The listing builds one solid part. Answer for the finished solid, in the listing's coordinates (mm). Face numbers are marked on the shaded views. A direction names the side the tool comes from. Coordinates: 2 decimals unless noted, no trailing zeros. Loops run counter-clockwise (first coordinate to the right, second up) from the corner with the lowest first, then second, coordinate; pieces in that order, holes last. Notation, with made-up numbers: M 6,-18 L 24,-18 A33 cw 24,11 Z; hole C -17,55.25 d6. An arc over 180 degrees is marked long. Answer in a Markdown table with one row per item. Add a question column.
from build123d import *

# Parameters (mm, degrees)
SKETCH001_W  = 155
SKETCH001_H  = 210
PAD_DEPTH    = 25
THICKNESS_T  = -0.5
SKETCH_W     = 30
SKETCH_H     = 13.5
PAD001_DEPTH = 5
FILLET_R     = 1
FILLET001_R  = 1


with BuildPart() as part:
    # Sketch001 → Pad (new body)
    with BuildSketch(Plane.XY):
        with Locations((77.5, 105)):
            Rectangle(SKETCH001_W, SKETCH001_H)
    extrude(amount=PAD_DEPTH)

    # Thickness
    thickness_openings = [part.faces().sort_by_distance(p)[0] for p in [
        (77.5, 105, 25),
    ]]
    offset(amount=THICKNESS_T, openings=thickness_openings)

    # Sketch → Pad001 (join)
    with BuildSketch(Plane.XY):
        with Locations((50, 105)):
            Rectangle(SKETCH_W, SKETCH_H)
        with Locations((105, 105)):
            Rectangle(SKETCH_W, SKETCH_H)
    extrude(amount=PAD001_DEPTH)

    # Fillet
    fillet_edges = [part.edges().sort_by_distance(p)[0] for p in [
        (77.5, 0.5, 0.5),
        (0.5, 105, 0.5),
        (154.5, 105, 0.5),
        (77.5, 209.5, 0.5),
        (50, 98.25, 0.5),
        (65, 105, 0.5),
        (50, 111.75, 0.5),
        (35, 105, 0.5),
        (120, 105, 0.5),
        (105, 111.75, 0.5),
        (90, 105, 0.5),
        (105, 98.25, 0.5),
    ]]
    fillet(fillet_edges, radius=FILLET_R)

    # Fillet001
    fillet001_edges = [part.edges().sort_by_distance(p)[0] for p in [
        (35, 105, 5),
        (50, 98.25, 5),
        (65, 105, 5),
        (50, 111.75, 5),
        (120, 105, 5),
        (105, 98.25, 5),
        (90, 105, 5),
        (105, 111.75, 5),
    ]]
    fillet(fillet001_edges, radius=FILLET001_R)


solid = part.part
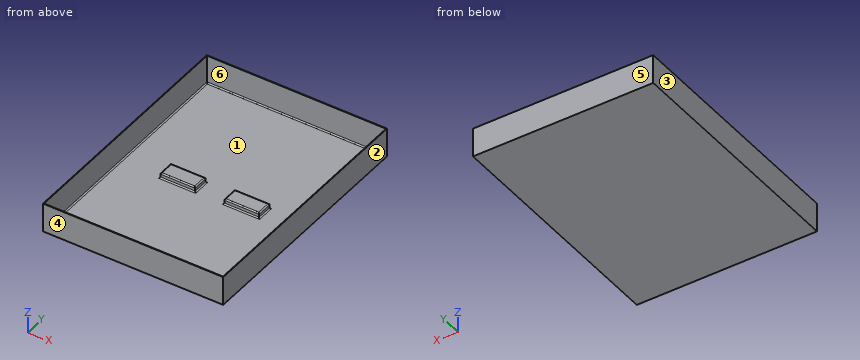
(1) Straight lines are drawn through the part: line 1 (X direction, y = 81, z = 2.5); line 2 (Y direction, x = 143, z = 10); line 3 (Z direction, x = 68, y = 117). For each, find the intervals that lie inside material, in ascending order.
(2) A cutting plane is placed at A-A (x = 47). Give the vertices of the cut face in (y, z).
(3) A cutting plane is placed at B-B (y = 108). Give the vertices of the cut face in (x, z), plus the area to 3 significant figures.
(4) A cutting plane is placed at D-D (x = 130). Give the vertices of the cut face in (y, z), plus the area to 3 significant figures.
(5) The mould has two halves that part along X. Classify the marked faces 1, 2, 3 and 4: released by +X, released by -X, zero draft, split by the parting line, or undercut.
(6) A cutting plane is placed at C-C (z = 13). Give the vertices of the cut face in (x, y).
(7) For the marked faces 5 and 6, determine the directions among +Z, -Z, +X, -X, +Y, -Y from which every point of the face is accessible in a straight line to the end or side of a thin tool.
(8) Each of these flat-tipped pins is pushed along its axis until it touches: pin 1 (1 mm diameter, centred on x = 121.5, y = 142.5, fed in from +Z); pin 2 (6 mm diameter, centred on x = 103, y = 102.5, fed in from +Z). Where does it stop, or does it pass through?
Solved:
| question | item | result |
|---|---|---|
| 1 | line 1 | x = 0 to 0.5, 154.5 to 155 |
| 1 | line 2 | y = 0 to 0.5, 209.5 to 210 |
| 1 | line 3 | z = 0 to 0.5 |
| 2 | outline | M 0,0 L 210,0 L 210,25 L 209.5,25 L 209.5,1.5 A1 cw 208.5,0.5 L 112.75,0.5 A1 cw 111.75,1.5 L 111.75,4 A1 ccw 110.75,5 L 99.25,5 A1 ccw 98.25,4 L 98.25,1.5 A1 cw 97.25,0.5 L 1.5,0.5 A1 cw 0.5,1.5 L 0.5,25 L 0,25 Z |
| 3 | outline | M 0,0 L 155,0 L 155,25 L 154.5,25 L 154.5,1.5 A1 cw 153.5,0.5 L 121,0.5 A1 cw 120,1.5 L 120,4 A1 ccw 119,5 L 91,5 A1 ccw 90,4 L 90,1.5 A1 cw 89,0.5 L 66,0.5 A1 cw 65,1.5 L 65,4 A1 ccw 64,5 L 36,5 A1 ccw 35,4 L 35,1.5 A1 cw 34,0.5 L 1.5,0.5 A1 cw 0.5,1.5 L 0.5,25 L 0,25 Z |
| 3 | area | 372 mm² |
| 4 | outline | M 0,0 L 210,0 L 210,25 L 209.5,25 L 209.5,1.5 A1 cw 208.5,0.5 L 1.5,0.5 A1 cw 0.5,1.5 L 0.5,25 L 0,25 Z |
| 4 | area | 130 mm² |
| 5 | face 1 | undercut |
| 5 | face 2 | released by +X |
| 5 | face 3 | released by -X |
| 5 | face 4 | zero draft |
| 6 | outline | M 0,0 L 155,0 L 155,210 L 0,210 Z; hole M 0.5,0.5 L 154.5,0.5 L 154.5,209.5 L 0.5,209.5 Z |
| 7 | face 5 | +Z, -Z, +X, -X, +Y |
| 7 | face 6 | +Z |
| 8 | pin 1 | stops at z = 0.5 |
| 8 | pin 2 | stops at z = 5 |
